Can you work these out from the drawing? Everything is in mm from the part's minimum corner. A direction names the side the tool comes from. Coordinates: 2 decimals unless noted, no trailing zeros. Order: outer loops, then holes, each group sorted by start corner. A loop starts at its lowest first (then second) coordinate and runs counter-clockwise, first axis right, second up. Notation, with made-up numbers: (61, 4) - (106, 4) arc R18 cw to (106, 20) - close; hole circle Ø4 at (-10.75, 58). An arc over 180 degrees is marked (long way). Use CSV: the item, a comma, the result in double quotes. Start each with the question number.
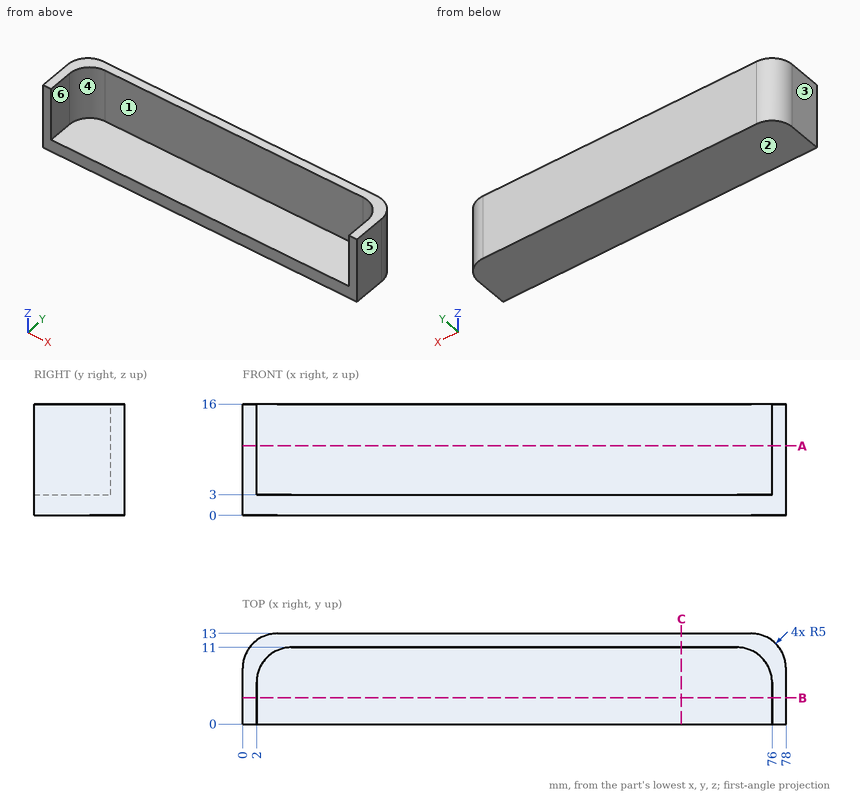
Item 1: For pin 1 Ø3 at (x, z) = (10.5, 5.5) entering from -Y; pin 2 Ø1.5 at (x, y) = (44, 7) entering from +Z; pin 3 Ø5 at (y, z) = (2.5, 11.5) entering from -X, each with a flat end and sliding along its axis, tell me the tip position at first contact or that it passes through.
Item 2: Suppose I cut it at C-C on x = 63. Write out the boundary of the cut face in (y, z).
Item 3: Suppose I cut it at B-B on y = 3.75. Write out the boundary of the cut face in (x, z), then the cut area to 3 significant figures.
Item 4: For the marked faces 5 and 6, which set-ups out of +Z, -Z, +X, -X, +Y, -Y let a thin tool reach every point of the face, with its end or its side?
Item 5: Suppose I cut it at A-A on z = 10. Write out the boundary of the cut face in (x, y), then the cut area to 3 significant figures.
Item 6: We'd pull the mould along X, two halves only. Please class the marked faces 1, 2, 3 and 4: released by +X, released by -X, zero draft, split by the parting line, or undercut.
Item 7: Please list where these lines run through material, in increasing order: line 1 along X through (y, z) = (5.25, 6); line 2 along Z through (x, y) = (41, 9.5); line 3 along Y through (x, z) = (69, 4). Write a range as from..to.
Here are the results:
1,pin 1,"y = 11"
1,pin 2,"z = 3"
1,pin 3,"x = 0"
2,outline,"(0, 0) - (13, 0) - (13, 16) - (11, 16) - (11, 3) - (0, 3) - close"
3,outline,"(0, 0) - (78, 0) - (78, 16) - (76, 16) - (76, 3) - (2, 3) - (2, 16) - (0, 16) - close"
3,area,"286 mm^2"
4,face 5,"+Z, -Z, +X, +Y, -Y"
4,face 6,"+Z, -Y"
5,outline,"(0, 0) - (2, 0) - (2, 6) arc R5 cw to (7, 11) - (71, 11) arc R5 cw to (76, 6) - (76, 0) - (78, 0) - (78, 8) arc R5 ccw to (73, 13) - (5, 13) arc R5 ccw to (0, 8) - close"
5,area,"200 mm^2"
6,face 1,"undercut"
6,face 2,"zero draft"
6,face 3,"released by -X"
6,face 4,"undercut"
7,line 1,"0..2, 76..78"
7,line 2,"0..3"
7,line 3,"11..13"
